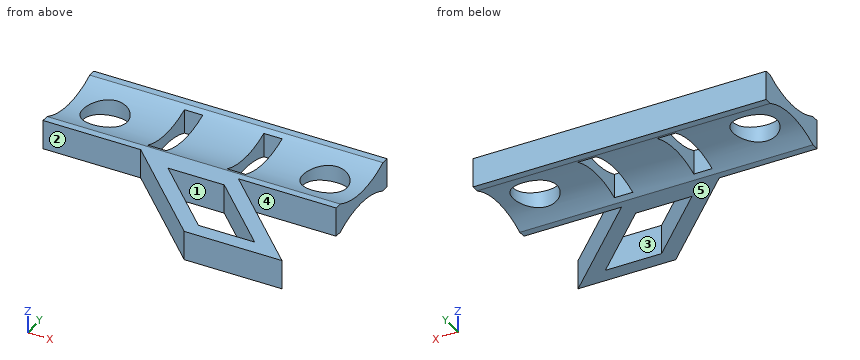
```python
from build123d import *

# Parameters (mm, degrees)
SKETCH_R     = 6
SKETCH_W     = 5
SKETCH_H     = 18
PAD_DEPTH    = 4
POCKET_DEPTH = 80.001


with BuildPart() as part:
    # Sketch → Pad (new body, symmetric)
    with BuildSketch(Plane.XY):
        Polygon((-40, 12.5), (-40, -12.5), (-13.333333, -12.5), (13.333333, -39.166667), (40, -39.166667), (13.333333, -12.5), (40, -12.5), (40, 12.5), align=None)
        with Locations((-30, 0)):
            Circle(SKETCH_R, mode=Mode.SUBTRACT)
        with Locations((30, 0)):
            Circle(SKETCH_R, mode=Mode.SUBTRACT)
        with Locations((-10.833333, 0)):
            Rectangle(SKETCH_W, SKETCH_H, mode=Mode.SUBTRACT)
        with Locations((10.833333, 0)):
            Rectangle(SKETCH_W, SKETCH_H, mode=Mode.SUBTRACT)
        Polygon((-3.676479, -16.5), (11.676479, -16.5), (30.343146, -35.166667), (14.990188, -35.166667), align=None, mode=Mode.SUBTRACT)
    extrude(amount=PAD_DEPTH, both=True)

    # Sketch002 → Pocket (cut, through all)
    with BuildSketch(Plane(origin=(-40, 0, 0), x_dir=(0, -1, 0), z_dir=(-1, 0, 0))):
        with BuildLine():
            ThreePointArc((-10.5, 4), (0, 1.5), (10.5, 4))
            Line((-10.5, 4), (10.5, 4))
        make_face()
        with BuildLine():
            Line((-10.5, -4), (10.5, -4))
            ThreePointArc((10.5, -4), (0, -1.5), (-10.5, -4))
        make_face()
    extrude(amount=-POCKET_DEPTH, mode=Mode.SUBTRACT)


solid = part.part
```
Input: part model. Units: mm. Frame: model coordinates. Face numbers are marked on the shaded views. A direction names the side the tool comes from. Round coordinates to 2 decimals unless told otherwise and drop trailing zeros. Loops run counter-clockwise (first coordinate to the right, second up) from the corner with the lowest first, then second, coordinate; pieces in that order, holes last. Notation, with made-up numbers: (44.25, -19) - (58.25, -19) arc R24 cw to (58.25, 8) - close; hole circle Ø8 at (21, -14.75). An arc over 180 degrees is marked (long way). One line per item, written item: value. Start each with the question number.
(1) Ray query, line 1 (X direction, y = 0, z = 0.55); line 2 (X direction, y = -8, z = -2); line 3 (Y direction, x = -30, z = -1.15). Return the intervals inside material, ascending. Write a range as [from, to].
(2) Section D-D, the plane y = -33. Return loops of the section in (x, z), plus the area to 3 significant figures.
(3) Section B-B, the plane x = -30. Return loops of the section in (y, z).
(4) Draft query along X for the marked faces 1 and 2. Return one class per face: +X half, -X half, draft (parallel to the pull), parting line (faces both ways), or undercut.
(5) Section A-A, the plane z = -0.5. Return loops of the section in (x, y), plus the area to 3 significant figures.
(6) Section C-C, the plane y = 0. Return loops of the section in (x, z), plus the area to 3 significant figures.
(7) Contact query for flat-ended pins moving along their axis: P1, Ø3, axis at y = -25.5, z = -3, coming from the +X side; P2, Ø3, axis at y = -23, z = -1.5, coming from the +X side; P3, Ø2.5, axis at x = -11.5, z = 1, coming from the -Y side. Output: stop coordinate, or through.
(8) Access query for the marked faces 3, 4 and 5. Directions: +Z, -Z, +X, -X, +Y, -Y. A direction counts if a zero-diameter tool reaches every point of the face in a straight line with its end or side. Return the directions, or none.
Results below:
1. line 1: [-40, -36], [-24, -13.33], [-8.33, 8.33], [13.33, 24], [36, 40]
1. line 2: [-40, -13.33], [-8.33, 8.33], [13.33, 40]
1. line 3: [-12.5, -6], [6, 12.5]
2. outline: (7.17, -4) - (12.82, -4) - (12.82, 4) - (7.17, 4) - close; (28.18, -4) - (33.83, -4) - (33.83, 4) - (28.18, 4) - close
2. area: 90.5 mm^2
3. outline: (-12.5, -4) - (-10.5, -4) arc R23.3 cw to (-6, -2.29) - (-6, 2.29) arc R23.3 cw to (-10.5, 4) - (-12.5, 4) - close; (6, -2.29) arc R23.3 cw to (10.5, -4) - (12.5, -4) - (12.5, 4) - (10.5, 4) arc R23.3 cw to (6, 2.29) - close
4. face 1: undercut
4. face 2: draft
5. outline: (-40, -12.5) - (-13.33, -12.5) - (13.33, -39.17) - (40, -39.17) - (13.33, -12.5) - (40, -12.5) - (40, 12.5) - (-40, 12.5) - close; hole circle Ø12 at (-30, 0); hole (-13.33, -9) - (-8.33, -9) - (-8.33, 9) - (-13.33, 9) - close; hole (-3.68, -16.5) - (14.99, -35.17) - (30.34, -35.17) - (11.68, -16.5) - close; hole (8.33, -9) - (13.33, -9) - (13.33, 9) - (8.33, 9) - close; hole circle Ø12 at (30, 0)
5. area: 2,020 mm^2
6. outline: (-40, -1.5) - (-36, -1.5) - (-36, 1.5) - (-40, 1.5) - close; (-24, -1.5) - (-13.33, -1.5) - (-13.33, 1.5) - (-24, 1.5) - close; (-8.33, -1.5) - (8.33, -1.5) - (8.33, 1.5) - (-8.33, 1.5) - close; (13.33, -1.5) - (24, -1.5) - (24, 1.5) - (13.33, 1.5) - close; (36, -1.5) - (40, -1.5) - (40, 1.5) - (36, 1.5) - close
6. area: 138 mm^2
7. P1: x = 27.83
7. P2: x = 25.33
7. P3: y = -15.58
8. face 3: +Z, -Z
8. face 4: +Z, -Z, +X
8. face 5: -Z, +X, -X, +Y, -Y
